Autodesk Inventor part; units mm, degrees
ref_plane "YZ Plane" through (0, 0, 0) normal (1, 0, 0) x (0, 1, 0)
ref_plane "XZ Plane" through (0, 0, 0) normal (0, 1, 0) x (-1, 0, 0)
ref_plane "XY Plane" through (0, 0, 0) normal (0, 0, 1) x (1, 0, 0)
sketch "Sketch1" plane through (0, 0, 0) normal (0, 0, 1) x (1, 0, 0)
  circle A0 centre (13.45, 22.5) radius 1.59
  circle A1 centre (2.35, 12.65) radius 1.59
  circle A2 centre (24.55, 2.35) radius 1.59
  line L0 (0, 0) -> (0, 15)
  line L1 (0, 15) -> (8.45, 15)
  line L2 (8.45, 15) -> (8.45, 27.5)
  line L3 (8.45, 27.5) -> (18.45, 27.5)
  line L4 (18.45, 27.5) -> (18.45, 15)
  line L5 (18.45, 15) -> (26.9, 15)
  line L6 (26.9, 15) -> (26.9, 0)
  line L7 (26.9, 0) -> (0, 0)
  point P0 (13.45, 27.5)
  dimension "d8" = 3.18
  dimension "d9" = 10.3
  dimension "d10" = 22.2
  dimension "d18" = 15
  dimension "d19" = 2.35
  dimension "d20" = 2.35
  dimension "d21" = 2.35
  dimension "d22" = 2.35
  dimension "d24" = 26.9
  dimension "d27" = 5
  dimension "d30" = 12.5
  dimension "d32" = 10
  dimension "d33" = 8.45
  dimension "d34" = 8.45
extrude "Extrusion1" add sketch "Sketch1" along normal blind 6.731
fillet "Fillet1" radius 1.5875 8 edges at (18.45, 15, 3.3655) (8.45, 15, 3.3655) (0, 0, 3.3655) (26.9, 0, 3.3655) (0, 15, 3.3655) (8.45, 27.5, 3.3655) (18.45, 27.5, 3.3655) (26.9, 15, 3.3655)
equation "\"d19\" = d22"
equation "\"d20\" = d19"
equation "\"d21\" = d19"
equation "\"d33\" = d34"
equation "\"d2\" = THICKB"
equation "\"THICKA\" = 3.175"
equation "\"THICKB\" = 6.731"
equation "\"THICKC\" = 12.7"
equation "\"BALLDIA\" = 12"
equation "\"MAGDIA\" = 9.5"
equation "\"THICKPLY\" = 5"
properties part number "EndStop_Bracket"
Design review of the part built by this model. Coordinates are the model's own, in mm. A direction names the side the tool comes from. Give positions to 0.01 mm unless a question says otherwise; leave off trailing zeros. Loops run counter-clockwise (first coordinate to the right, second up) from the corner with the lowest first, then second, coordinate; pieces in that order, holes last. Notation, with made-up numbers: (5.5, -7.5) -> (51.5, -7.5) arc R17 ccw to (51.5, -2.5) -> close; hole circle Ø7 at (-8.5, -34.75). An arc over 180 degrees is marked (long way). One line per question, with ' | ' between items. Start each with the question number.
(1) Draft analysis for pull direction X (two halves, no side actions). For faces 3 (the face through (18.9, 15.48, 3.41)), 4 (the face through (7.97, 15.45, 3.41)), 5 (the face through (14.2, 23.9, 3.3)), state which applies: +X half, -X half, draft (parallel to the pull), parting line (faces both ways), or undercut.
(2) We need section A-A (x = 2.35). State the section outline as (y, z) points.
(3) We need section B-B (z = 6). State how many separate pieces and enclosed holes the cut face has, and give its area (3 significant figures).
(4) For faces 1 (the face through (0.45, 0.48, 3.41)), 2 (the face through (4, 15, 3)), list the 3-axis set-ups (+Z, -Z, +X, -X, +Y, -Y) from which the entire face can be reached by the end or side of a thin tool; tool diameter is ignored.
(5) We need section D-D (y = 17). State the section outline as (x, z) points, and give its area (3 significant figures).
(6) Insertion check: P1, Ø3.5, axis at x = 2.35, y = 12.65, coming from the -Z side; P2, Ø2.5, axis at x = 5, z = 3.5, coming from the +Y side; P3, Ø2, axis at y = 14.5, z = 2.5, coming from the -X side; P4, Ø2, axis at y = 23, z = 4.5, coming from the -X side. Each pin has a flat end and moves straight along its axis. Give the tip position at first contact, or say it passes through.
(7) We need section C-C (y = 22.5). State the section outline as (x, z) points, and give its area (3 significant figures).
(8) For line 1 (Y direction, x = 24.55, z = 1.75); line 2 (X direction, y = 25.25, z = 5); line 3 (Y direction, x = 13.45, z = 1.5), list the stretches that pass through material, from the lowest coordinate up.
The answers:
1) face 3: +X half | face 4: -X half | face 5: undercut
2) outline: (0, 0) -> (11.06, 0) -> (11.06, 6.73) -> (0, 6.73) -> close; (14.24, 0) -> (15, 0) -> (15, 6.73) -> (14.24, 6.73) -> close
3) separate pieces: 1 | enclosed holes: 3 | area: 503 mm^2
4) face 1: +Z, -Z, -X, -Y | face 2: +Z, -Z, -X, +Y
5) outline: (8.45, 0) -> (18.45, 0) -> (18.45, 6.73) -> (8.45, 6.73) -> close | area: 67.3 mm^2
6) P1: stops at z = 0 | P2: stops at y = 15 | P3: stops at x = 0 | P4: stops at x = 8.45
7) outline: (8.45, 0) -> (11.86, 0) -> (11.86, 6.73) -> (8.45, 6.73) -> close; (15.04, 0) -> (18.45, 0) -> (18.45, 6.73) -> (15.04, 6.73) -> close | area: 45.9 mm^2
8) line 1: y = 0 to 0.76, 3.94 to 15 | line 2: x = 8.45 to 18.45 | line 3: y = 0 to 20.91, 24.09 to 27.5
